Check sheet for the modelled part. Datum: model origin and axes. Units: mm. A direction names the side the tool comes from. Give positions to 0.01 mm unless a question says otherwise; leave off trailing zeros. Order: outer loops, then holes, each group sorted by start corner. A loop starts at its lowest first (then second) coordinate and runs counter-clockwise, first axis right, second up.
Item 1: Access from +Z, -Z, +X, -X, +Y, -Y to the whole of each face (thin tool, end or side, straight path). Record for faces 5 (the flat face through (-31.692, 0.356, 34.944)), 6 (the flat face through (-52.243, 0, 25)), 7 (the flat face through (-38.46, 0.17, 40.46)).
Item 2: Sectioned sample at C-C on z = 15. Record the boundary of the cut face in (x, y).
Item 3: Release check for a two-part mould opening along Y. For faces 1 (the flat face through (-37.988, 8.77, 41.886)), 2 (the flat face through (-38, 9.987, 20)), 3 (the flat face through (-23.243, 0, 16)), 4 (the cylindrical face through (-24.92, -0.19, 33.69)) record: released by +Y, released by -Y, zero draft, split by the parting line, or undercut.
Item 4: Sectioned sample at D-D on y = 8.75. Record the boundary of the cut face in (x, z).
Item 5: Sectioned sample at B-B on x = -47. Record the boundary of the cut face in (y, z).
Item 6: Material ranges on line 1 along X through (y, z) = (0.25, 20); line 2 along Y through (x, z) = (-42.5, 37.5); line 3 along X through (y, z) = (-4, 33.5), recorded low to high.
Item 7: Gauge pin test, flat ends, axial feed: P1, Ø1.8, axis at x = -34.35, y = 0.26, coming from the +Z side; P2, Ø1, axis at y = 3.5, z = 34.5, coming from the +X side; P3, Ø2, axis at x = -32.5, y = -3, coming from the +Z side; P4, Ø2, axis at x = -34.5, y = 2, coming from the -Z side. Record the tip position at first contact, or that the pin passes through.
from build123d import *

# Parameters (mm, degrees)
F0_W     = 35
F0_H     = 19.45
F0_W_2   = 29
F0_H_2   = 13.45
F1_DEPTH = 51.5
F3_DEPTH = 25
F4_W     = 16.598594
F4_H     = 13.45
F4_R     = 1.5
F5_DEPTH = 3
F6_R     = 1.5
F7_DEPTH = 46.3


with BuildPart() as f1:
    # F0 (on Top) → F1 (new body)
    with BuildSketch(Plane.XY):
        with Locations((-37.743293, 0.261565)):
            Rectangle(F0_W, F0_H)
        with Locations((-37.743293, 0.261565)):
            Rectangle(F0_W_2, F0_H_2, mode=Mode.SUBTRACT)
    extrude(amount=F1_DEPTH)

    # F2 (on face) → F3 (cut)
    with BuildSketch(Plane.XZ.offset(9.463435)):
        Polygon((-20.243293, 51.5), (-55.243293, 51.5), (-20.243293, 32), align=None)
    extrude(amount=-F3_DEPTH, mode=Mode.SUBTRACT)

    # F4 (on face) → F5 (join)
    with BuildSketch(Plane(origin=(8.810147, 0, 15.813084), x_dir=(0.873568, 0, -0.486702), z_dir=(0.486702, 0, 0.873568))):
        with Locations((-44.99185, 0.261565)):
            Rectangle(F4_W, F4_H)
        with Locations((-49.282474, 0.261565)):
            Circle(F4_R, mode=Mode.SUBTRACT)
        with Locations((-41.720062, 0)):
            Circle(F4_R, mode=Mode.SUBTRACT)
        Polygon((-35.897397, 6.986565), (-36.692553, 6.986565), (-36.692553, -6.463435), (-35.849709, -6.463435), align=None)
        with Locations((-41.720062, 0)):
            Circle(F4_R)
        with Locations((-49.282474, 0.261565)):
            Circle(F4_R)
    extrude(amount=-F5_DEPTH)

    # F6 (on face) → F7 (cut)
    with BuildSketch(Plane(origin=(0, 0, 0), x_dir=(1, 0, 0), z_dir=(0, 0, -1))):
        with Locations((-26.34857, -0.261565)):
            Circle(F6_R)
        with Locations((-34.34857, -0.261565)):
            Circle(F6_R)
    extrude(amount=-F7_DEPTH, mode=Mode.SUBTRACT)


solid = f1.part
Report:
1. face 5: -Z
1. face 6: +Z, -Z
1. face 7: +Z
2. outline: (-55.24, -9.46) - (-20.24, -9.46) - (-20.24, 9.99) - (-55.24, 9.99) - close; hole (-52.24, -6.46) - (-23.24, -6.46) - (-23.24, 6.99) - (-52.24, 6.99) - close
3. face 1: zero draft
3. face 2: released by +Y
3. face 3: undercut
3. face 4: undercut
4. outline: (-55.24, 0) - (-20.24, 0) - (-20.24, 32) - (-55.24, 51.5) - close
5. outline: (-9.46, 0) - (-6.46, 0) - (-6.46, 46.91) - (-9.46, 46.91) - close; (6.99, 0) - (9.99, 0) - (9.99, 46.91) - (6.99, 46.91) - close
6. line 1: x = -55.24 to -52.24, -23.24 to -20.24
6. line 2: y = -9.46 to -6.46, 6.99 to 9.99
6. line 3: x = -55.24 to -52.24, -29.1 to -22.94
7. P1: passes through
7. P2: stops at x = -23.83
7. P3: stops at z = 39.39
7. P4: stops at z = 35.95
